from build123d import *

# Parameters (mm, degrees)
SKETCH1_R           = 7.5
BOSS_EXTRUDE1_DEPTH = 81.44


with BuildPart() as part:
    # Sketch1 → Boss-Extrude1 (new body)
    with BuildSketch(Plane.XY):
        with BuildLine():
            Line((-20.35, 14), (20.35, 14))
            Line((20.35, 14), (20.35, 8))
            Line((20.35, 8), (14, 8))
            Line((14, 8), (14, 0))
            ThreePointArc((14, 0), (0, -14), (-14, 0))
            Line((-14, 0), (-14, 8))
            Line((-14, 8), (-20.35, 8))
            Line((-20.35, 8), (-20.35, 14))
        make_face()
        Circle(SKETCH1_R, mode=Mode.SUBTRACT)
    extrude(amount=BOSS_EXTRUDE1_DEPTH)


solid = part.part
Input: part model. Units: mm. Frame: model coordinates. A direction names the side the tool comes from. Give positions to 0.01 mm unless a question says otherwise; leave off trailing zeros. Loops run counter-clockwise (first coordinate to the right, second up) from the corner with the lowest first, then second, coordinate; pieces in that order, holes last. Notation, with made-up numbers: M -8,51 L 15,51 A18 ccw 15,59 Z; hole C 38,23 d3. An arc over 180 degrees is marked long. Use one line per item in the form item = value.
1. Section query A-A, the plane x = 0. Return the cut outline in (y, z).
Numbers:
outline = M -14,0 L -7.5,0 L -7.5,81.44 L -14,81.44 Z; M 7.5,0 L 14,0 L 14,81.44 L 7.5,81.44 Z
2. Section query B-B, the plane z = 64.5. Return the cut outline in (x, y).
Numbers:
outline = M -20.35,8 L -14,8 L -14,0 A14 ccw 14,0 L 14,8 L 20.35,8 L 20.35,14 L -20.35,14 Z; hole C 0,0 d15
3. Section query C-C, the plane y = 5.75. Return the cut outline in (x, z), and give its area (3 significant figures).
Numbers:
outline = M -14,0 L -4.82,0 L -4.82,81.44 L -14,81.44 Z; M 4.82,0 L 14,0 L 14,81.44 L 4.82,81.44 Z
area = 1,500 mm²
4. First-contact query: pin 1 (4 mm diameter, centred on y = 0.5, z = 27.5, fed in from +X); pin 2 (5 mm diameter, centred on x = -17, z = 36, fed in from -Y); pin 3 (5 mm diameter, centred on x = -6.5, z = 30, fed in from -Y). Flat tips, straight axial feed; report the tip coordinate or a pass-through.
Numbers:
pin_1 = 14
pin_2 = 8
pin_3 = -13.42
5. Section query D-D, the plane x = 17. Return the cut outline in (y, z).
Numbers:
outline = M 8,0 L 14,0 L 14,81.44 L 8,81.44 Z
6. Reachability of faces 1 (the face through (-4.2, 6.4, 0)), 2 (the face through (-14, 4, 40)), 3 (the face through (17, 8, 40)) from +Z, -Z, +X, -X, +Y, -Y: full face, straight path, thin tool, end or side. Return the list, or none.
Numbers:
face_1 = -Z, +X, -X, +Y, -Y
face_2 = +Z, -Z, -X, -Y
face_3 = +Z, -Z, +X, -Y
7. Line query: L1, parallel to Y at x = 0, z = 34; L2, parallel to Y at x = -6, z = 35; L3, parallel to X at y = -4, z = 4. Output: solid intervals per line, ascending.
Numbers:
L1 = -14 to -7.5, 7.5 to 14
L2 = -12.65 to -4.5, 4.5 to 14
L3 = -13.42 to -6.34, 6.34 to 13.42
8. Pull-direction query (X, two-part tool) for faces 4 (the face through (-7.493, 0.33, 40.15)), 5 (the face through (20.35, 11, 40)), 6 (the face through (0, 14, 40)); classes: released by +X, released by -X, zero draft, split by the parting line, or undercut.
Numbers:
face_4 = undercut
face_5 = released by +X
face_6 = zero draft
